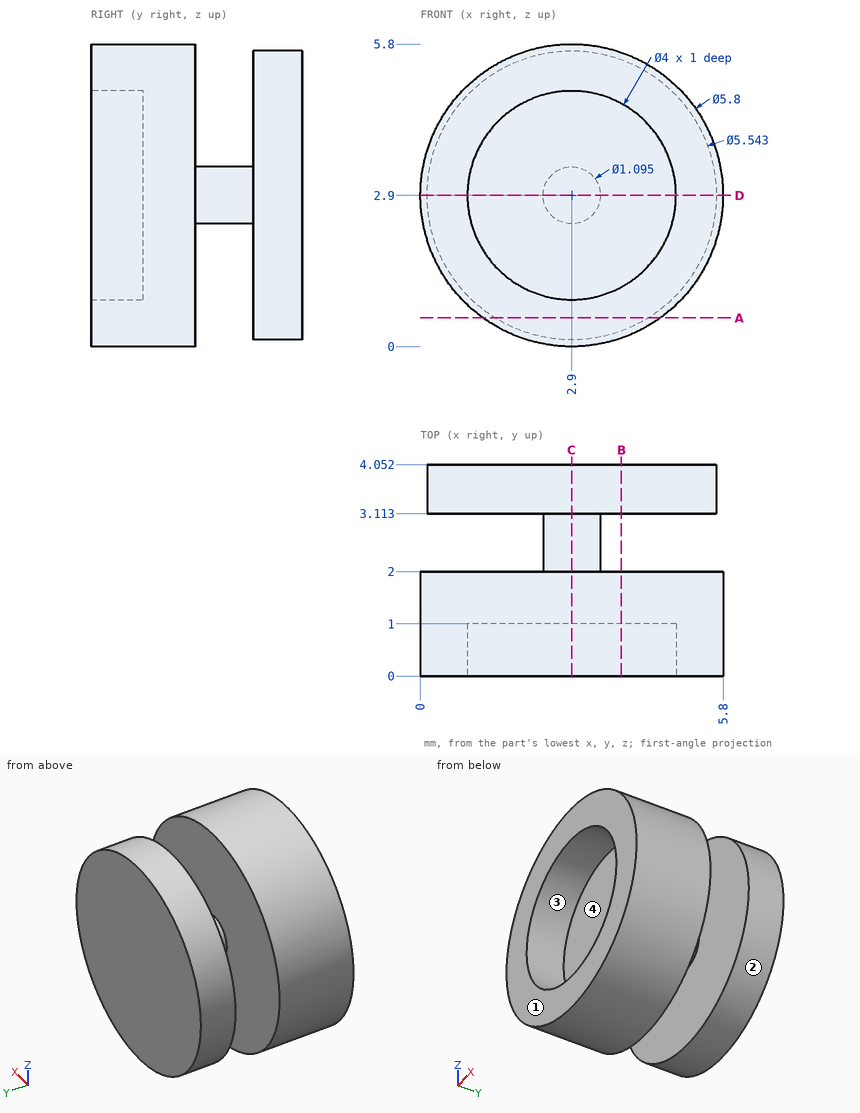
Verification items for this drawing (mm, ordinates from the low corner). Give positions to 0.01 mm unless a question says otherwise; leave off trailing zeros. Write each loop counter-clockwise with the first axis right and the second up, starting at its lowest first coordinate (ties: lowest second). Pieces come first, ordered by that corner, then holes. Notation, with made-up numbers: (-33.5, -33) - (-3.5, -33) arc R16 cw to (-3.5, -25) - close; hole circle Ø10 at (87.5, -25.5). An arc over 180 degrees is marked (long way). Answer as CSV lines item,"result". Start each with the question number.
1. Sectioned sample at C-C (x = 2.9). Record the boundary of the cut face in (y, z), then the cut area to 3 significant figures.
2. Sectioned sample at B-B (x = 3.85). Record the boundary of the cut face in (y, z).
3. Sectioned sample at A-A (z = 0.55). Record the boundary of the cut face in (x, y).
4. Draft check along Z on the marked faces 1, 2, 3 and 4. Enter one of: pulls with the +Z half, pulls with the -Z half, needs draft (parallel to the pull), parting line crosses it, or undercut.
5. Sectioned sample at D-D (z = 2.9). Record the boundary of the cut face in (x, y).
6. Depth check by flat-ended pin: pin 1 (2 mm diameter, centred on x = 4.5, y = 1.5, fed in from -Z); pin 2 (1 mm diameter, centred on x = 2.5, y = 3.5, fed in from +Z); pin 3 (1.5 mm diameter, centred on y = 1.5, z = 4.5, fed in from +X). Enter the tip coordinate at first touch or a pass-through.
7. Thickness scan on line 1 (Y direction, x = 1.8, z = 1.95); line 2 (X direction, y = 0.7, z = 2.9); line 3 (Y direction, x = 5, z = 3.7). Record the ranges inside material, lowest first.
Derived:
1,outline,"(0, 0) - (2, 0) - (2, 2.35) - (3.11, 2.35) - (3.11, 0.13) - (4.05, 0.13) - (4.05, 5.67) - (3.11, 5.67) - (3.11, 3.45) - (2, 3.45) - (2, 5.8) - (0, 5.8) - (0, 4.9) - (1, 4.9) - (1, 0.9) - (0, 0.9) - close"
1,area,"14.0 mm²"
2,outline,"(0, 0.16) - (2, 0.16) - (2, 5.64) - (0, 5.64) - (0, 4.66) - (1, 4.66) - (1, 1.14) - (0, 1.14) - close; (3.11, 0.3) - (4.05, 0.3) - (4.05, 5.5) - (3.11, 5.5) - close"
3,outline,"(1.2, 0) - (4.6, 0) - (4.6, 2) - (1.2, 2) - close; (1.43, 3.11) - (4.37, 3.11) - (4.37, 4.05) - (1.43, 4.05) - close"
4,face 1,"needs draft"
4,face 2,"parting line crosses it"
4,face 3,"undercut"
4,face 4,"undercut"
5,outline,"(0, 0) - (0.9, 0) - (0.9, 1) - (4.9, 1) - (4.9, 0) - (5.8, 0) - (5.8, 2) - (3.45, 2) - (3.45, 3.11) - (5.67, 3.11) - (5.67, 4.05) - (0.13, 4.05) - (0.13, 3.11) - (2.35, 3.11) - (2.35, 2) - (0, 2) - close"
6,pin 1,"z = 0.06"
6,pin 2,"z = 5.67"
6,pin 3,"x = 5.67"
7,line 1,"1 to 2, 3.11 to 4.05"
7,line 2,"0 to 0.9, 4.9 to 5.8"
7,line 3,"0 to 2, 3.11 to 4.05"
